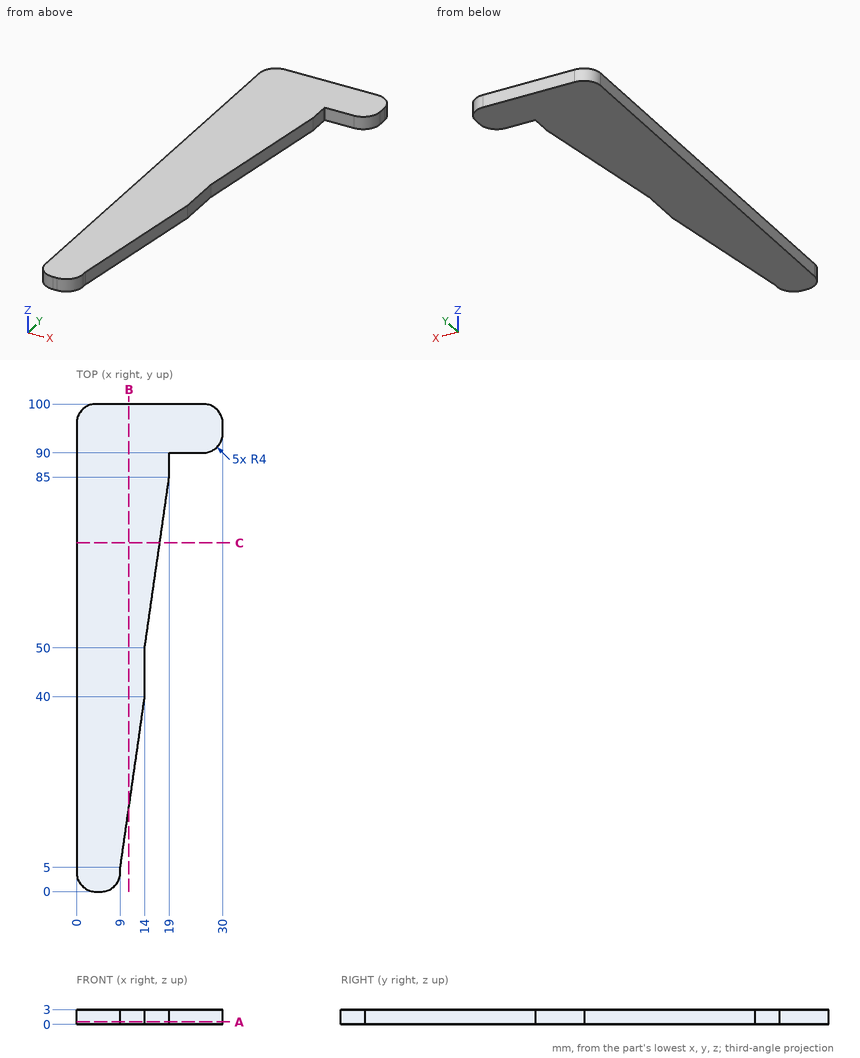
Verification items for this drawing (mm, ordinates from the low corner). Coordinates: 2 decimals unless noted, no trailing zeros. Write each loop counter-clockwise with the first axis right and the second up, starting at its lowest first coordinate (ties: lowest second). Pieces come first, ordered by that corner, then holes. Notation, with made-up numbers: (-8.5, 42.5) -> (0.5, 42.5) arc R25 cw to (0.5, 57.5) -> close; hole circle Ø10 at (-4, 45.5). An arc over 180 degrees is marked (long way). One line per item, written item: value. Start each with the question number.
Q1. Cross-section at A-A on z = 0.5. Enter the section's corners in (x, y), and give its area (3 significant figures).
Q2. Thickness scan on L1, parallel to Y at x = 25.5, z = 1.7; L2, parallel to X at y = 46, z = 0.55; L3, parallel to X at y = 86, z = 0.35. Record the ranges inside material, lowest first. Write a range as from..to.
Q3. Cross-section at C-C on y = 71.5. Enter the section's corners in (x, z), and give its area (3 significant figures).
Q4. Cross-section at B-B on x = 10.75. Enter the section's corners in (y, z), and give its area (3 significant figures).
Q5. Go/stop test with flat-tipped pins: P1, Ø1, axis at x = 21, z = 1.5, coming from the -Y side; P2, Ø0.8, axis at y = 4.5, z = 1, coming from the +X side. Record where each tip stops, or that it passes through.
Checked values:
1. outline: (0, 4) arc R4 ccw to (4, 0) -> (5, 0) arc R4 ccw to (9, 4) -> (9, 5) -> (14, 40) -> (14, 50) -> (19, 85) -> (19, 90) -> (26, 90) arc R4 ccw to (30, 94) -> (30, 96) arc R4 ccw to (26, 100) -> (4, 100) arc R4 ccw to (0, 96) -> close
1. area: 1,540 mm²
2. L1: y = 90..100
2. L2: x = 0..14
2. L3: x = 0..19
3. outline: (0, 0) -> (17.07, 0) -> (17.07, 3) -> (0, 3) -> close
3. area: 51.2 mm²
4. outline: (17.25, 0) -> (100, 0) -> (100, 3) -> (17.25, 3) -> close
4. area: 248 mm²
5. P1: stops at y = 90
5. P2: stops at x = 9
